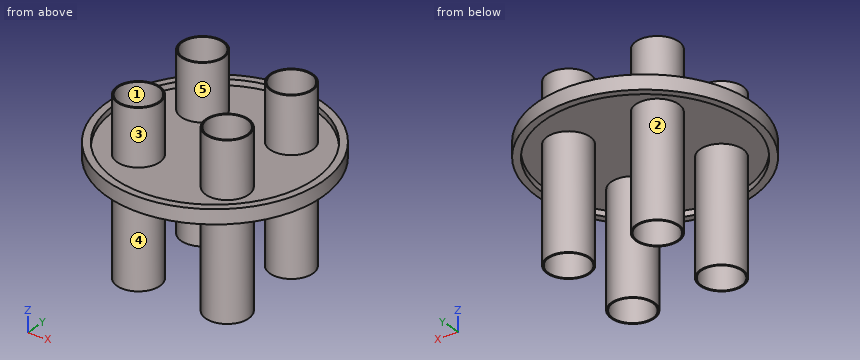
from build123d import *

# Parameters (mm, degrees)
BOSS_EXTRUDE1_DEPTH      = 2.5
BOSS_EXTRUDE1_DEPTH_BACK = 2.5
SKETCH1_R                = 37.5
SKETCH1_R_2              = 35
BOSS_EXTRUDE2_DEPTH      = 0.5
BOSS_EXTRUDE2_DEPTH_BACK = 0.5
SKETCH1_3_R              = 35
SKETCH1_3_R_2            = 7.5
SKETCH1_3_R_3            = 2.5
BOSS_EXTRUDE3_DEPTH      = 20
BOSS_EXTRUDE3_DEPTH_BACK = 40
SKETCH1_4_R              = 7.5
SKETCH1_4_R_2            = 7


with BuildPart() as part:
    # Sketch1 → Boss-Extrude1 (new, two sides: drawn at the far end of the back side and taken through both)
    with BuildSketch(Plane.XY.offset(-BOSS_EXTRUDE1_DEPTH_BACK)):
        Circle(SKETCH1_R)
        Circle(SKETCH1_R_2, mode=Mode.SUBTRACT)
    extrude(amount=BOSS_EXTRUDE1_DEPTH + BOSS_EXTRUDE1_DEPTH_BACK)

    # Sketch1<3> → Boss-Extrude2 (add, two sides: drawn at the far end of the back side and taken through both)
    with BuildSketch(Plane.XY.offset(-BOSS_EXTRUDE2_DEPTH_BACK)):
        Circle(SKETCH1_3_R)
        with Locations((-15.384748909, -15.487184505)):
            Circle(SKETCH1_3_R_2, mode=Mode.SUBTRACT)
        with Locations((15.487184505, -15.384748909)):
            Circle(SKETCH1_3_R_2, mode=Mode.SUBTRACT)
        with Locations((15.384748909, 15.487184505)):
            Circle(SKETCH1_3_R_2, mode=Mode.SUBTRACT)
        with Locations((-15.487184505, 15.384748909)):
            Circle(SKETCH1_3_R_2, mode=Mode.SUBTRACT)
        Circle(SKETCH1_3_R_3, mode=Mode.SUBTRACT)
    extrude(amount=BOSS_EXTRUDE2_DEPTH + BOSS_EXTRUDE2_DEPTH_BACK)

    # Sketch1<4> → Boss-Extrude3 (add, two sides: drawn at the far end of the back side and taken through both)
    # profile 1 of 4: a face of its own
    with BuildSketch(Plane.XY.offset(-BOSS_EXTRUDE3_DEPTH_BACK)):
        with Locations((-15.487184505, 15.384748909)):
            Circle(SKETCH1_4_R)
        with Locations((-15.487184505, 15.384748909)):
            Circle(SKETCH1_4_R_2, mode=Mode.SUBTRACT)
    # profile 2 of 4: a face of its own
    with BuildSketch(Plane.XY.offset(-BOSS_EXTRUDE3_DEPTH_BACK)):
        with Locations((15.384748909, 15.487184505)):
            Circle(SKETCH1_4_R)
        with Locations((15.384748909, 15.487184505)):
            Circle(SKETCH1_4_R_2, mode=Mode.SUBTRACT)
    # profile 3 of 4: a face of its own
    with BuildSketch(Plane.XY.offset(-BOSS_EXTRUDE3_DEPTH_BACK)):
        with Locations((15.487184505, -15.384748909)):
            Circle(SKETCH1_4_R)
        with Locations((15.487184505, -15.384748909)):
            Circle(SKETCH1_4_R_2, mode=Mode.SUBTRACT)
    # profile 4 of 4: a face of its own
    with BuildSketch(Plane.XY.offset(-BOSS_EXTRUDE3_DEPTH_BACK)):
        with Locations((-15.384748909, -15.487184505)):
            Circle(SKETCH1_4_R)
        with Locations((-15.384748909, -15.487184505)):
            Circle(SKETCH1_4_R_2, mode=Mode.SUBTRACT)
    extrude(amount=BOSS_EXTRUDE3_DEPTH + BOSS_EXTRUDE3_DEPTH_BACK)


solid = part.part
Build history of the part. All positions in model axes, mm. Face numbers are marked on the shaded views. A direction names the side the tool comes from. Round coordinates to 2 decimals unless told otherwise and drop trailing zeros. Write each loop counter-clockwise with the first axis right and the second up, starting at its lowest first coordinate (ties: lowest second). Pieces come first, ordered by that corner, then holes. Notation, with made-up numbers: M -10,-12.5 L 26,-12.5 A27 cw 26,26.5 Z; hole C 4.25,-2.75 d11. An arc over 180 degrees is marked long. Answer as a JSON object with one key per item and string values. Group by question number.
(1) Mould opens along X. For the marked faces 4 and 5 say: pulls with the +X half, pulls with the -X half, needs draft (parallel to the pull), parting line crosses it, or undercut.
(2) Drill centre lines: L1, parallel to Y at x = -15, z = -25; L2, parallel to Y at x = 19, z = 6.5; L3, parallel to Y at x = 19.5, z = -1.5. Where is each one in solid material? Low to high.
(3) Cut at D-D (y = 24.5). Give the cut face in (x, z) (3 decimals).
(4) Flat gauge pins, fed straight in: pin 1 (1.5 mm diameter, centred on x = 17, y = 1, fed in from -Z); pin 2 (22.5 mm diameter, centred on x = -15.49, y = 15.38, fed in from +Z); pin 3 (10 mm diameter, centred on x = 18.5, z = -14.5, fed in from +Y); pin 4 (1 mm diameter, centred on x = 23.5, y = 28.5, fed in from -Z). Where does each tip first touch, or does it go through?
(5) Cut at A-A (y = 0). Give the cut face in (x, z), and give its area (3 significant figures).
(6) Which spindle directions (+Z, -Z, +X, -X, +Y, -Y) get a long thin tool onto all of the face, cutting with end or side? Do the marked faces 1, 2 and 3. Say none if no direction does.
(7) Cut at C-C (z = 12). Give the cut face in (x, y), and give its area (3 significant figures).
Responses:
{
 "1": {"face 4": "undercut", "face 5": "undercut"},
 "2": {"L1": "y = -22.98 to -22.48, -8.5 to -8, 7.9 to 8.4, 22.37 to 22.87", "L2": "y = -22.01 to -21.44, -9.33 to -8.76, 8.92 to 9.49, 21.48 to 22.06", "L3": "y = -32.03 to -29.06, -21.72 to -21.12, -9.65 to -9.05, 9.22 to 9.82, 21.15 to 21.76, 29.06 to 32.03"},
 "3": {"outline": "M -28.39,-2.5 L -24.995,-2.5 L -24.995,-0.5 L 24.995,-0.5 L 24.995,-2.5 L 28.39,-2.5 L 28.39,2.5 L 24.995,2.5 L 24.995,0.5 L -24.995,0.5 L -24.995,2.5 L -28.39,2.5 Z"},
 "4": {"pin 1": "stops at z = -0.5", "pin 2": "stops at z = 20", "pin 3": "stops at y = 22.99", "pin 4": "stops at z = -2.5"},
 "5": {"outline": "M -37.5,-2.5 L -35,-2.5 L -35,-0.5 L -2.5,-0.5 L -2.5,0.5 L -35,0.5 L -35,2.5 L -37.5,2.5 Z; M 2.5,-0.5 L 35,-0.5 L 35,-2.5 L 37.5,-2.5 L 37.5,2.5 L 35,2.5 L 35,0.5 L 2.5,0.5 Z", "area": "90.0 mm2"},
 "6": {"face 1": "+Z, -Z", "face 2": "-Z", "face 3": "+Z"},
 "7": {"outline": "C -15.49,15.38 d15; C -15.38,-15.49 d15; C 15.38,15.49 d15; C 15.49,-15.38 d15; hole C -15.49,15.38 d14; hole C -15.38,-15.49 d14; hole C 15.38,15.49 d14; hole C 15.49,-15.38 d14", "area": "91.1 mm2"}
}
